from build123d import *

# Parameters (mm, degrees)
F0_W     = 54
F0_H     = 84
F1_DEPTH = 6
F3_R     = 2
F4_DEPTH = 6


with BuildPart() as f1:
    # F0 (on Top) → F1 (new body)
    with BuildSketch(Plane.XY):
        Rectangle(F0_W, F0_H)
    extrude(amount=F1_DEPTH)

    # F3 (on face) → F4 (cut, through all)
    with BuildSketch(Plane.XY.offset(6)):
        with Locations((-7.5, 14)):
            Circle(F3_R)
        with Locations((-7.5, -14)):
            Circle(F3_R)
        with Locations((-20, 5)):
            Circle(F3_R)
        with Locations((-20, -5)):
            Circle(F3_R)
        with Locations((21, 14)):
            Circle(F3_R)
        with Locations((21, -14)):
            Circle(F3_R)
        with Locations((21, -35)):
            Circle(F3_R)
        with Locations((21, 35)):
            Circle(F3_R)
        with Locations((-20, 37)):
            Circle(F3_R)
        with Locations((-7.5, 35)):
            Circle(F3_R)
        with Locations((-20, -37)):
            Circle(F3_R)
        with Locations((-7.5, -35)):
            Circle(F3_R)
    extrude(amount=-F4_DEPTH, mode=Mode.SUBTRACT)


solid = f1.part
The listing builds one solid part. Answer for the finished solid, in the listing's coordinates (mm). Give positions to 0.01 mm unless a question says otherwise; leave off trailing zeros. Write each loop counter-clockwise with the first axis right and the second up, starting at its lowest first coordinate (ties: lowest second). Pieces come first, ordered by that corner, then holes. Notation, with made-up numbers: (86, 58) -> (129, 58) arc R27 ccw to (129, 74) -> close; hole circle Ø5 at (17, 60). An arc over 180 degrees is marked (long way). One line per question, with ' | ' between items. Start each with the question number.
1. Section B-B (x = 21) is taken. Determine the outline of the cut face in (y, z).
2. Section C-C (y = -14) is taken. Determine the outline of the cut face in (x, z), plus the area to 3 significant figures.
3. For a pull along X with two mould halves and no side action, classify faces 1 (the flat face through (27, -1, 3)), 2 (the flat face through (-27, -1, 3)), 3 (the flat face through (0, -42, 3)), 4 (the cylindrical face through (-7.934, -36.952, 3.042)) as pulls with the +X half, pulls with the -X half, needs draft (parallel to the pull), parting line crosses it, or undercut.
4. Section D-D (z = 4.1) is taken. State how many separate pieces and enclosed holes the cut face has, plus the area to 3 significant figures.
5. Find the intervals of material crossed by probe 1 along Y at (x, z) = (-20, 3.25); probe 2 along Y at (x, z) = (21, 3); probe 3 along X at (y, z) = (15, 1.15), in increasing order.
6. Section A-A (y = -5) is taken. Determine the outline of the cut face in (x, z).
7. Given pin 1 Ø2.5 at (x, y) = (-7.5, 35) entering from +Z, flat-ended and moving along its own axis, determine where the tip first touches the part or whether it passes through.
Response values:
1) outline: (-42, 0) -> (-37, 0) -> (-37, 6) -> (-42, 6) -> close; (-33, 0) -> (-16, 0) -> (-16, 6) -> (-33, 6) -> close; (-12, 0) -> (12, 0) -> (12, 6) -> (-12, 6) -> close; (16, 0) -> (33, 0) -> (33, 6) -> (16, 6) -> close; (37, 0) -> (42, 0) -> (42, 6) -> (37, 6) -> close
2) outline: (-27, 0) -> (-9.5, 0) -> (-9.5, 6) -> (-27, 6) -> close; (-5.5, 0) -> (19, 0) -> (19, 6) -> (-5.5, 6) -> close; (23, 0) -> (27, 0) -> (27, 6) -> (23, 6) -> close | area: 276 mm2
3) face 1: pulls with the +X half | face 2: pulls with the -X half | face 3: needs draft | face 4: undercut
4) separate pieces: 1 | enclosed holes: 12 | area: 4,390 mm2
5) probe 1: -42 to -39, -35 to -7, -3 to 3, 7 to 35, 39 to 42 | probe 2: -42 to -37, -33 to -16, -12 to 12, 16 to 33, 37 to 42 | probe 3: -27 to -9.23, -5.77 to 19.27, 22.73 to 27
6) outline: (-27, 0) -> (-22, 0) -> (-22, 6) -> (-27, 6) -> close; (-18, 0) -> (27, 0) -> (27, 6) -> (-18, 6) -> close
7) pin 1: through
